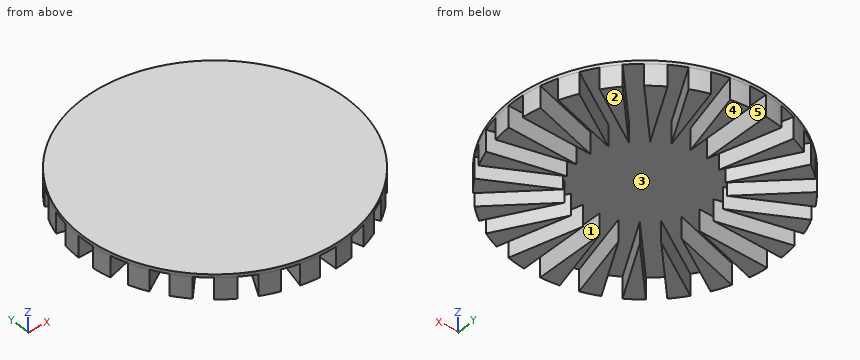
```python
from build123d import *

# Parameters (mm, degrees)
BOSS_EXTRUDE1_START = 13
SKETCH1_R           = 80
BOSS_EXTRUDE1_DEPTH = 2
BOSS_EXTRUDE2_START = -15
BOSS_EXTRUDE2_DEPTH = 15
CIRPATTERN1_COUNT   = 24


with BuildPart() as part:
    # Sketch1 → Boss-Extrude1 (new body)
    with BuildSketch(Plane.XY.offset(BOSS_EXTRUDE1_START)):
        Circle(SKETCH1_R)
    extrude(amount=BOSS_EXTRUDE1_DEPTH)

    # Sketch3 → Boss-Extrude2 (add)
    with BuildSketch(Plane.XY.offset(15).offset(BOSS_EXTRUDE2_START)):
        with BuildLine():
            Line((-5, -79.843597113), (-5, -37.978770564))
            Line((-5, -37.978770564), (-15.835414431, -78.417087741))
            ThreePointArc((-15.835414431, -78.417087741), (-10.442095378, -79.31558891), (-5, -79.843597113))
        make_face()
    boss_extrude2 = extrude(amount=BOSS_EXTRUDE2_DEPTH)

    # CirPattern1: Boss-Extrude2 ×24 about axis
    cirpattern1_axis = Axis((0, 0, 0), (0, 0, 1))
    for i in range(1, CIRPATTERN1_COUNT):
        add(boss_extrude2.rotate(cirpattern1_axis, i * 360 / CIRPATTERN1_COUNT))


solid = part.part
```
Input: part model. Units: mm. Frame: model coordinates. Face numbers are marked on the shaded views. A direction names the side the tool comes from. Round coordinates to 2 decimals unless told otherwise and drop trailing zeros. Loops run counter-clockwise (first coordinate to the right, second up) from the corner with the lowest first, then second, coordinate; pieces in that order, holes last. Notation, with made-up numbers: M 86.5,45 L 92.5,45 A13 cw 92.5,63 Z; hole C 3,76 d5. An arc over 180 degrees is marked long. Answer in a Markdown table with one row per item. Add a question column.
1. Section B-B (y = 33). Output: boundary loops of the cut face in (x, z), and give its area (3 significant figures).
2. Contact query for flat-ended pins moving along their axis: pin 1 (6.5 mm diameter, centred on x = -52.5, z = 6, fed in from -Y); pin 2 (4 mm diameter, centred on y = -54.5, z = 9, fed in from -X); pin 3 (6.5 mm diameter, centred on x = 51, z = 6, fed in from -Y). Output: stop coordinate, or through.
3. Section D-D (y = 63). Output: boundary loops of the cut face in (x, z).
4. Section C-C (x = 0). Output: boundary loops of the cut face in (y, z), and give its area (3 significant figures).
5. Mould query, pull axis X, two halves, no side actions, for the marked faces 3, 4 and 5. Classes: released by +X, released by -X, zero draft, split by the parting line, or undercut.
6. Set-up query: the marked faces 1 and 2. Return all of +Z, -Z, +X, -X, +Y, -Y with unobstructed straight access to the full face (end or side cutting, diameter ignored); none if empty.
7. Ray query, probe 1 along X at (y, z) = (-28.5, 6.5); probe 2 along X at (y, z) = (-67, 11); probe 3 along Y at (x, z) = (29, 9.5). Return the intervals inside material, ascending.
8. Section A-A (z = 9.5). Give the number of separate pieces and of enclosed holes in the cut face, and give its area (3 significant figures).
Values follow:
| question | item | result |
|---|---|---|
| 1 | outline | M -72.88,0 L -67.16,0 L -67.16,13 L -47.16,13 L -47.16,0 L -40.07,0 L -40.07,13 L -25.93,13 L -25.93,0 L -24.83,0 L -24.83,13 L 24.83,13 L 24.83,0 L 25.93,0 L 25.93,13 L 40.07,13 L 40.07,0 L 47.16,0 L 47.16,13 L 67.16,13 L 67.16,0 L 72.88,0 L 72.88,15 L -72.88,15 Z |
| 1 | area | 653 mm^2 |
| 2 | pin 1 | y = -63.04 |
| 2 | pin 2 | x = -60.36 |
| 2 | pin 3 | y = -64.19 |
| 3 | outline | M -49.31,0 L -42.15,0 L -42.15,13 L -30.6,13 L -30.6,0 L -22.06,0 L -22.06,13 L -11.7,13 L -11.7,0 L -5,0 L -5,13 L 5,13 L 5,0 L 11.7,0 L 11.7,13 L 22.06,13 L 22.06,0 L 30.6,0 L 30.6,13 L 42.15,13 L 42.15,0 L 49.31,0 L 49.31,15 L -49.31,15 Z |
| 4 | outline | M -80,13 L 80,13 L 80,15 L -80,15 Z |
| 4 | area | 320 mm^2 |
| 5 | face 3 | undercut |
| 5 | face 4 | zero draft |
| 5 | face 5 | undercut |
| 6 | face 1 | -Z, +Y, -Y |
| 6 | face 2 | -Z, +X, -X, +Y, -Y |
| 7 | probe 1 | -74.75 to -59.36, -39.36 to -35.57, 35.57 to 39.36, 59.36 to 74.75 |
| 7 | probe 2 | -32.91 to -23.13, -12.78 to -5, 5 to 12.78, 23.13 to 32.91 |
| 7 | probe 3 | -74.56 to -60.23, -40.23 to -36.07, 36.07 to 40.23, 60.23 to 74.56 |
| 8 | separate pieces | 24 |
| 8 | enclosed holes | 0 |
| 8 | area | 5,480 mm^2 |
